Read the model definition and answer for the solid it produces. Units are mm, in the model's axes. Coordinates: 2 decimals unless noted, no trailing zeros. Write each loop counter-clockwise with the first axis right and the second up, starting at its lowest first coordinate (ties: lowest second). Pieces come first, ordered by that corner, then holes.
(1) Straight lines are drawn through the part: line 1 along Z through (x, y) = (19, 1.8); line 2 along Z through (x, y) = (17, 1.4). For each, find the intervals that lie inside material, in ascending order.
(2) The part is cut by section C-C, the plane z = 0. Determine the outline of the cut face in (x, y).
(3) The part is cut by section B-B, the plane x = 0. Determine the outline of the cut face in (y, z), and give its area (3 significant figures).
(4) Given pin 1 (0.6 mm diameter, centred on x = -24.5, y = 1.5, fed in from -Z); pin 2 (1 mm diameter, centred on y = 1.5, z = 9, fed in from +X), each flat-ended and moving along its own axis, determine where each tip first touches the part or whether it passes through.
```python
from build123d import *

# Parameters (mm, degrees)
ESQUISSE1_R                  = 25.95
BOSS_EXTRU_1_DEPTH           = 2
ENL_V_MAT_EXTRU_8_DEPTH      = 2
R_P_TITION_CIRCULAIRE1_COUNT = 4


with BuildPart() as part:
    # Esquisse1 → Boss.-Extru.1 (new body)
    with BuildSketch(Plane(origin=(0, 0, 0), x_dir=(1, 0, 0), z_dir=(0, 1, 0))):
        with Locations(Location((0, 0, 0), (0, 0, 270))):  # turned: the seam where the file's is
            Circle(ESQUISSE1_R)
    extrude(amount=BOSS_EXTRU_1_DEPTH)

    # Esquisse2 → Enlèv. mat.-Extru.8 (cut)
    with BuildSketch(Plane(origin=(0, 0, 0), x_dir=(1, 0, 0), z_dir=(0, 1, 0))):
        with BuildLine():
            Line((-1.55, 25.903667694), (-1.55, 23.55))
            ThreePointArc((-1.55, 23.55), (0, 22), (1.55, 23.55))
            Line((1.55, 23.55), (1.55, 25.903667694))
            ThreePointArc((1.55, 25.903667694), (0, 25.95), (-1.55, 25.903667694))
        make_face()
        with BuildLine():
            Line((8.160057781, 24.633634669), (6.917968061, 20.884006271))
            ThreePointArc((6.917968061, 20.884006271), (11, 19.052558883), (14.627095933, 16.433139219))
            Line((14.627095933, 16.433139219), (17.253324521, 19.383634669))
            ThreePointArc((17.253324521, 19.383634669), (12.975, 22.473359228), (8.160057781, 24.633634669))
        make_face()
    enl_v_mat_extru_8 = extrude(amount=ENL_V_MAT_EXTRU_8_DEPTH, mode=Mode.SUBTRACT)

    # Répétition circulaire1: Enlèv. mat.-Extru.8 ×4 about axis
    r_p_tition_circulaire1_axis = Axis((0, 0, 0), (0, 1, 0))
    for i in range(1, R_P_TITION_CIRCULAIRE1_COUNT):
        add(enl_v_mat_extru_8.rotate(r_p_tition_circulaire1_axis, i * 360 / R_P_TITION_CIRCULAIRE1_COUNT), mode=Mode.SUBTRACT)


solid = part.part
```
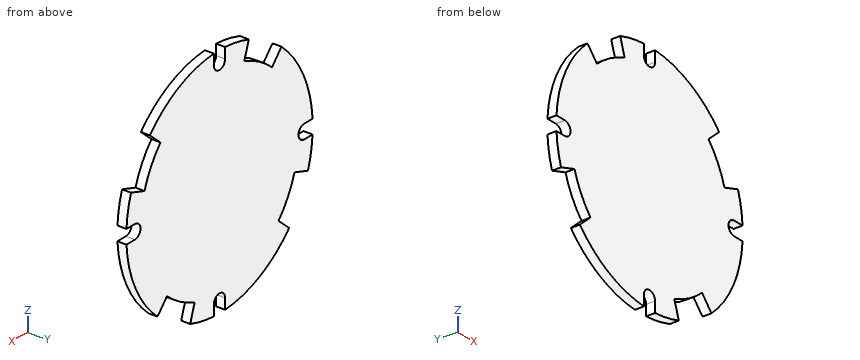
Computed:
1. line 1: z = -17.67 to 11.09, 16.91 to 17.67
1. line 2: z = -19.1 to 13.96, 15.13 to 19.61
2. outline: (-22, 0) - (22, 0) - (22, 2) - (-22, 2) - close
3. outline: (0, -22) - (2, -22) - (2, 22) - (0, 22) - close
3. area: 88.0 mm2
4. pin 1: stops at z = -8.16
4. pin 2: stops at x = 20.29
